Could you check a few things on this drawing? It's one solid part, dimensions in mm from its lowest x, y, z. Give positions to 0.01 mm unless a question says otherwise; leave off trailing zeros. Loops run counter-clockwise (first coordinate to the right, second up) from the corner with the lowest first, then second, coordinate; pieces in that order, holes last.
1. For P1, Ø1, axis at y = 6, z = 1.5, coming from the +X side; P2, Ø1, axis at y = 5.5, z = 4.5, coming from the -X side, each with a flat end and sliding along its axis, tell me the tip position at first contact or that it passes through.
2. Imagine slicing it at B-B (z = 2.7). List the corners of the cut face in (x, y) for me, plus the area to 3 significant figures.
3. Thinking about a two-plate mould opening in Y: for the marked faces 1, 2 and 3, which applies, +Y half, -Y half, draft (parallel to the pull), parting line (faces both ways), or undercut?
4. I need wall thicknesses on line 1 along Z through (x, y) = (2.7, 5.5); line 2 along X through (y, z) = (2.5, 2.85); line 3 along X through (y, z) = (6.75, 3.4). Which ranges of each line are inside material? Lowest first, please.
5. Imagine slicing it at A-A (x = 2.7). List the corners of the cut face in (y, z) for me, plus the area to 3 significant figures.
6. Imagine slicing it at C-C (y = 1.25). List the corners of the cut face in (x, z) for me, plus the area to 3 significant figures.
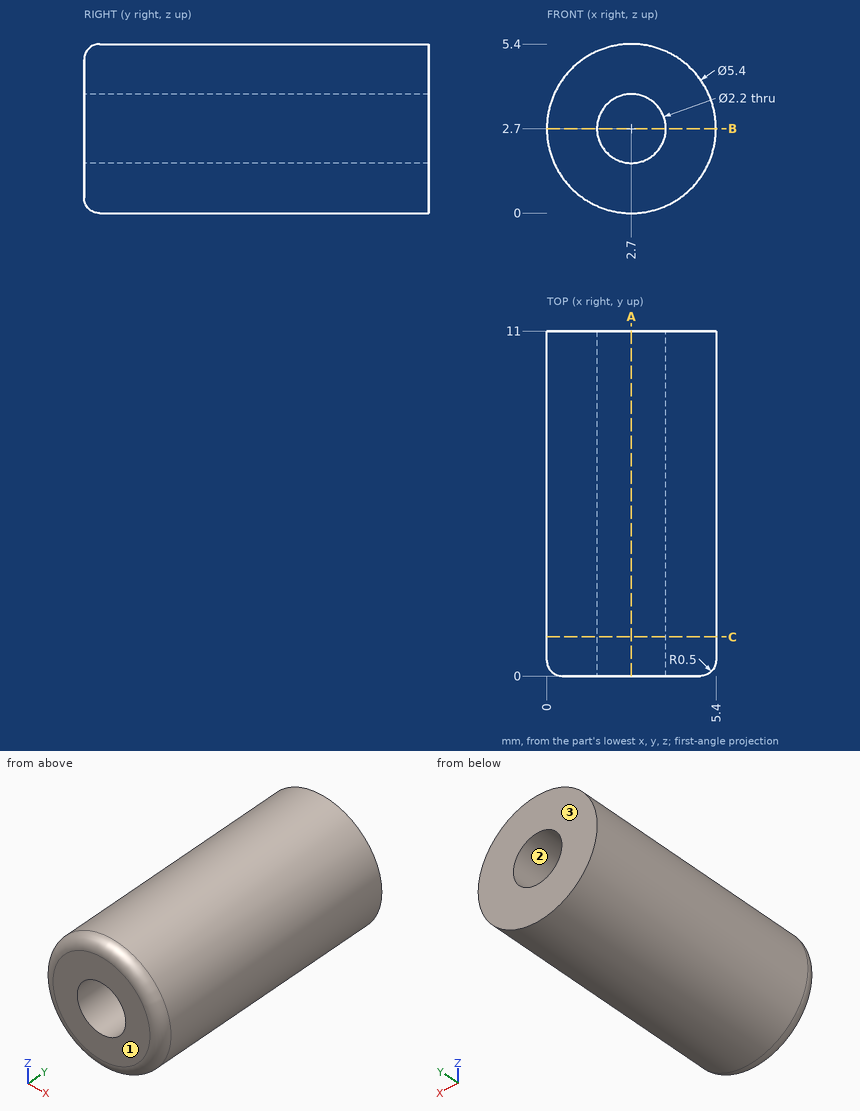
Derived:
1. P1: stops at x = 5.31
1. P2: stops at x = 0.33
2. outline: (0, 0.5) arc R0.5 ccw to (0.5, 0) - (1.6, 0) - (1.6, 11) - (0, 11) - close; (3.8, 0) - (4.9, 0) arc R0.5 ccw to (5.4, 0.5) - (5.4, 11) - (3.8, 11) - close
2. area: 35.1 mm2
3. face 1: -Y half
3. face 2: draft
3. face 3: +Y half
4. line 1: z = 0 to 1.6, 3.8 to 5.4
4. line 2: x = 0 to 1.61, 3.79 to 5.4
4. line 3: x = 0.09 to 1.85, 3.55 to 5.31
5. outline: (0, 0.5) arc R0.5 ccw to (0.5, 0) - (11, 0) - (11, 1.6) - (0, 1.6) - close; (0, 3.8) - (11, 3.8) - (11, 5.4) - (0.5, 5.4) arc R0.5 ccw to (0, 4.9) - close
5. area: 35.1 mm2
6. outline: circle Ø5.4 at (2.7, 2.7); hole circle Ø2.2 at (2.7, 2.7)
6. area: 19.1 mm2
